Geometry check sheet. Reference: the model listing, model coordinates, mm. Face numbers are marked on the shaded views. A direction names the side the tool comes from. Round coordinates to 2 decimals unless told otherwise and drop trailing zeros. Order: outer loops, then holes, each group sorted by start corner. A loop starts at its lowest first (then second) coordinate and runs counter-clockwise, first axis right, second up. Notation, with made-up numbers: (85.25, 77) - (125.25, 77) arc R34 ccw to (125.25, 113) - close; hole circle Ø9 at (30, 89.5). An arc over 180 degrees is marked (long way). Write each question's results on one line, items separated by ' | '.
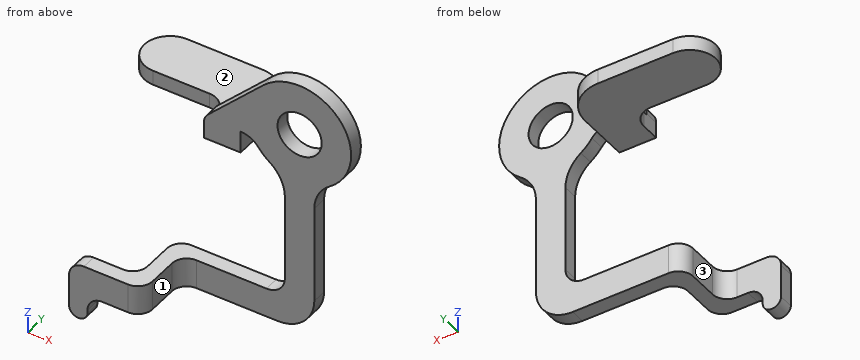
```python
from build123d import *

# Parameters (mm, degrees)
CROQUIS1_R              = 3
SALIENTE_EXTRUIR1_DEPTH = 2
SALIENTE_EXTRUIR2_DEPTH = 2
REDONDEO1_R             = 5
REDONDEO2_R             = 2.5
REDONDEO3_R             = 5
REDONDEO4_R             = 5
REDONDEO5_R             = 2
REDONDEO6_R             = 5
REDONDEO7_R             = 2.5
SALIENTE_EXTRUIR3_DEPTH = 4
REDONDEO8_R             = 2
REDONDEO9_R             = 2
SALIENTE_EXTRUIR4_DEPTH = 2
REDONDEO10_R            = 2
CORTAR_EXTRUIR1_DEPTH   = 2


with BuildPart() as part:
    # Croquis1 → Saliente-Extruir1 (new body)
    with BuildSketch(Plane(origin=(0, 0, 0), x_dir=(1, 0, 0), z_dir=(0, 1, 0))):
        with BuildLine():
            Line((2, 16.626040067), (2, 6.708203932))
            ThreePointArc((2, 6.708203932), (6.023877075, -3.56551609), (-4.918618823, -4.980681567))
            Line((-4.918618823, -4.980681567), (-13, 3))
            Line((-13, 3), (-13, 4))
            Line((-13, 4), (-8, 4))
            Line((-8, 4), (-8, 3))
            ThreePointArc((-8, 3), (-6.658359214, 3.316718427), (-5.6, 4.2))
            ThreePointArc((-5.6, 4.2), (-4.001596149, 5.743450902), (-2, 6.708203932))
            Line((-2, 6.708203932), (-2, 24))
            Line((-2, 24), (-16, 24))
            Line((-16, 24), (-16, 28))
            Line((-16, 28), (2, 28))
            Line((2, 28), (2, 16.626040067))
        make_face()
        Circle(CROQUIS1_R, mode=Mode.SUBTRACT)
    extrude(amount=SALIENTE_EXTRUIR1_DEPTH)

    # Croquis2 → Saliente-Extruir2 (add)
    with BuildSketch(Plane(origin=(0, 0, -4), x_dir=(-1, 0, 0), z_dir=(0, 0, -1))):
        with BuildLine():
            Line((8, 2), (8, 12))
            Line((8, 12), (23.192528099, 12))
            ThreePointArc((23.192528099, 12), (26.692528099, 8.5), (23.192528099, 5))
            Line((23.192528099, 5), (13, 5))
            Line((13, 5), (13, 2))
            Line((13, 2), (13, 0))
            Line((13, 0), (8, 0))
            Line((8, 0), (8, 2))
        make_face()
    extrude(amount=SALIENTE_EXTRUIR2_DEPTH)

    # Redondeo1
    redondeo1_edges = [part.edges().sort_by_distance(p)[0] for p in [
        (-8, 12, -5),
    ]]
    fillet(redondeo1_edges, radius=REDONDEO1_R)

    # Redondeo2
    redondeo2_edges = [part.edges().sort_by_distance(p)[0] for p in [
        (-13, 5, -5),
    ]]
    fillet(redondeo2_edges, radius=REDONDEO2_R)

    # Redondeo3
    redondeo3_edges = [part.edges().sort_by_distance(p)[0] for p in [
        (2, 1, -6.708203932),
    ]]
    fillet(redondeo3_edges, radius=REDONDEO3_R)

    # Redondeo4
    redondeo4_edges = [part.edges().sort_by_distance(p)[0] for p in [
        (-2, 1, -6.708203932),
    ]]
    fillet(redondeo4_edges, radius=REDONDEO4_R)

    # Redondeo5
    redondeo5_edges = [part.edges().sort_by_distance(p)[0] for p in [
        (-13, 1, -3),
    ]]
    fillet(redondeo5_edges, radius=REDONDEO5_R)

    # Redondeo6
    redondeo6_edges = [part.edges().sort_by_distance(p)[0] for p in [
        (2, 1, -28),
    ]]
    fillet(redondeo6_edges, radius=REDONDEO6_R)

    # Redondeo7
    redondeo7_edges = [part.edges().sort_by_distance(p)[0] for p in [
        (-2, 1, -24),
    ]]
    fillet(redondeo7_edges, radius=REDONDEO7_R)

    # Croquis3 → Saliente-Extruir3 (add)
    with BuildSketch(Plane(origin=(0, 0, -28), x_dir=(-1, 0, 0), z_dir=(0, 0, -1))):
        with BuildLine():
            Line((16, 2), (16, 0))
            Line((16, 0), (16, -6))
            ThreePointArc((16, -6), (16.585786438, -7.414213562), (18, -8))
            Line((18, -8), (26, -8))
            Line((26, -8), (26, -6))
            Line((26, -6), (18, -6))
            Line((18, -6), (18, 0))
            ThreePointArc((18, 0), (17.414213562, 1.414213562), (16, 2))
        make_face()
    extrude(amount=-SALIENTE_EXTRUIR3_DEPTH)

    # Redondeo8
    redondeo8_edges = [part.edges().sort_by_distance(p)[0] for p in [
        (-18, -6, -26),
    ]]
    fillet(redondeo8_edges, radius=REDONDEO8_R)

    # Redondeo9
    redondeo9_edges = [part.edges().sort_by_distance(p)[0] for p in [
        (-16, 0, -26),
    ]]
    fillet(redondeo9_edges, radius=REDONDEO9_R)

    # Croquis4 → Saliente-Extruir4 (add)
    with BuildSketch(Plane(origin=(0, -6, 0), x_dir=(1, 0, 0), z_dir=(0, 1, 0))):
        with BuildLine():
            Line((-23.5, 28), (-23.5, 30.5))
            ThreePointArc((-23.5, 30.5), (-24.75, 31.677994798), (-26, 30.5))
            Line((-26, 30.5), (-26, 28))
            Line((-26, 28), (-23.5, 28))
        make_face()
    extrude(amount=-SALIENTE_EXTRUIR4_DEPTH)

    # Redondeo10
    redondeo10_edges = [part.edges().sort_by_distance(p)[0] for p in [
        (-23.5, -7, -28),
    ]]
    fillet(redondeo10_edges, radius=REDONDEO10_R)

    # Croquis5 → Cortar-Extruir1 (cut)
    with BuildSketch(Plane(origin=(0, -6, 0), x_dir=(1, 0, 0), z_dir=(0, 1, 0))):
        with BuildLine():
            Line((-26, 24), (-26, 26))
            ThreePointArc((-26, 26), (-25.414213562, 24.585786438), (-24, 24))
            Line((-24, 24), (-26, 24))
        make_face()
    extrude(amount=-CORTAR_EXTRUIR1_DEPTH, mode=Mode.SUBTRACT)


solid = part.part
```
(1) Material ranges on line 1 (Y direction, x = -5, z = 3.5); line 2 (X direction, y = 1.4, z = 0); line 3 (Z direction, x = -24, y = 6.5), recorded low to high.
Answers follow:
line 1: 0 to 2 | line 2: -9.96 to -3, 3 to 7 | line 3: -6 to -4
(2) Access from +Z, -Z, +X, -X, +Y, -Y to the whole of each face (thin tool, end or side, straight path). Record for the marked faces 1, 2 and 3.
Answers follow:
face 1: +Z, -Z, +X, -Y | face 2: +Z, +X, -X, +Y | face 3: +Z, -Z, -X, +Y
(3) Section check B-B (z = 1.5). Record the cut outline in (x, y), then the cut area to 3 significant figures.
Answers follow:
outline: (-8.44, 0) - (-2.6, 0) - (-2.6, 2) - (-8.44, 2) - close; (2.6, 0) - (6.84, 0) - (6.84, 2) - (2.6, 2) - close | area: 20.2 mm²
(4) Section check C-C (y = 1). Record the cut outline in (x, z).
Answers follow:
outline: (-17.73, -28) - (-3, -28) arc R5 ccw to (2, -23) - (2, -9.75) arc R5 cw to (4.08, -5.69) arc R7 ccw (long way) to (-4.92, 4.98) - (-12.41, -2.41) arc R2 ccw to (-13, -3.84) - (-13, -6) - (-8, -6) - (-8, -3) arc R3 cw to (-5.6, -4.2) arc R7 ccw to (-4.08, -5.69) arc R5 cw to (-2, -9.75) - (-2, -21.5) arc R2.5 cw to (-4.5, -24) - (-17.73, -24) - close; hole circle Ø6 at (0, 0)
(5) Section check A-A (x = -13.5). Record the cut outline in (y, z).
Answers follow:
outline: (0, -28) - (2, -28) - (2, -24) - (0, -24) - close; (4, -6) - (12, -6) - (12, -4) - (4, -4) - close
(6) Section check D-D (z = -13.5). Record the cut outline in (x, y), then the cut area to 3 significant figures.
Answers follow:
outline: (-2, 0) - (2, 0) - (2, 2) - (-2, 2) - close | area: 8.00 mm²
(7) Depth check by flat-ended pin: pin 1 Ø3 at (x, y) = (-20.5, 8.5) entering from +Z; pin 2 Ø6.5 at (x, z) = (-22.5, -27.5) entering from +Y; pin 3 Ø1 at (x, z) = (-10.5, -5) entering from -Y; pin 4 Ø5 at (x, y) = (-8, -3) entering from -Z. Enter the tip coordinate at first touch or a pass-through.
Answers follow:
pin 1: z = -4 | pin 2: y = -5.85 | pin 3: y = 0 | pin 4: through
